Could you check a few things on this model? Use its own coordinates, in mm. A direction names the side the tool comes from. Round coordinates to 2 decimals unless told otherwise and drop trailing zeros. Write each loop counter-clockwise with the first axis right and the second up, starting at its lowest first coordinate (ties: lowest second). Pieces come first, ordered by that corner, then holes.
```python
from build123d import *

# Parameters (mm, degrees)
SKETCH1_W           = 54
SKETCH1_H           = 42
BOSS_EXTRUDE1_DEPTH = 40
BOSS_EXTRUDE2_DEPTH = 54
SKETCH12_W          = 20
SKETCH12_H          = 65.765371804
CUT_EXTRUDE5_DEPTH  = 157.508433956
SKETCH13_W          = 20
SKETCH13_H          = 20
CUT_EXTRUDE6_DEPTH  = 157.508433956
SKETCH14_W          = 7.9
SKETCH14_H          = 7.9
CUT_EXTRUDE7_DEPTH  = 20.2
BOSS_EXTRUDE3_DEPTH = 54
CUT_EXTRUDE8_DEPTH  = 54


with BuildPart() as part:
    # Sketch1 → Boss-Extrude1 (new body)
    with BuildSketch(Plane.XY):
        with Locations((27, 21)):
            Rectangle(SKETCH1_W, SKETCH1_H)
    extrude(amount=BOSS_EXTRUDE1_DEPTH)

    # Sketch5 → Boss-Extrude2 (add)
    with BuildSketch(Plane.ZY):
        Polygon((140.765371804, 42), (40, 42), (40, 0), (140.765371804, 27), align=None)
    extrude(amount=-BOSS_EXTRUDE2_DEPTH)

    # Sketch12 → Cut-Extrude5 (cut, through all)
    with BuildSketch(Plane(origin=(0, 42, 0), x_dir=(1, 0, 0), z_dir=(0, 1, 0))):
        with Locations((27, -67.882685902)):
            Rectangle(SKETCH12_W, SKETCH12_H)
    extrude(amount=-CUT_EXTRUDE5_DEPTH, mode=Mode.SUBTRACT)

    # Sketch13 → Cut-Extrude6 (cut, through all)
    with BuildSketch(Plane(origin=(0, 0, 0), x_dir=(-1, 0, 0), z_dir=(0, 0, -1))):
        with Locations((-27, 21)):
            Rectangle(SKETCH13_W, SKETCH13_H)
    extrude(amount=-CUT_EXTRUDE6_DEPTH, mode=Mode.SUBTRACT)

    # Sketch14 → Cut-Extrude7 (cut)
    with BuildSketch(Plane(origin=(0, 0, 0), x_dir=(-1, 0, 0), z_dir=(0, 0, -1))):
        with Locations((-45.25, 33.25)):
            Rectangle(SKETCH14_W, SKETCH14_H)
        with Locations((-45.25, 8.75)):
            Rectangle(SKETCH14_W, SKETCH14_H)
        with Locations((-8.75, 33.25)):
            Rectangle(SKETCH14_W, SKETCH14_H)
        with Locations((-8.75, 8.75)):
            Rectangle(SKETCH14_W, SKETCH14_H)
    extrude(amount=-CUT_EXTRUDE7_DEPTH, mode=Mode.SUBTRACT)

    # Sketch16 → Boss-Extrude3 (add)
    with BuildSketch(Plane(origin=(54, 0, 0), x_dir=(0, 0, -1), z_dir=(1, 0, 0))):
        Polygon((-140.765371804, 42), (-135.475562383, 72), (-87.112319758, 66.620193825), (-91.4535242, 42), align=None)
    extrude(amount=-BOSS_EXTRUDE3_DEPTH)

    # Sketch18 → Cut-Extrude8 (cut)
    with BuildSketch(Plane(origin=(54, 0, 0), x_dir=(0, 0, -1), z_dir=(1, 0, 0))):
        Polygon((-126.406728237, 70.991205567), (-135.475562383, 72), (-138.97204162, 52.170480871), (-121.632853281, 50.323309926), (-121.080075246, 55.292659626), (-126.9167299, 66.017283743), align=None)
        Polygon((-97.584499975, 67.785092966), (-98.201251534, 62.823277017), (-106.251724868, 53.643191009), (-106.804502902, 48.673841309), (-90.622534666, 46.712775836), (-87.112319758, 66.620193825), align=None)
    extrude(amount=-CUT_EXTRUDE8_DEPTH, mode=Mode.SUBTRACT)


solid = part.part
```
Q1. We'd pull the mould along Z, two halves only. Please class faces 5 (the flat face through (4.8, 33, 10)), 6 (the flat face through (27.378, 51.193, 106.524)), 7 (the flat face through (27, 37, 100.765)): pulls with the +Z half, pulls with the -Z half, needs draft (parallel to the pull), parting line crosses it, or undercut.
Q2. Imagine slicing it at D-D, the plane x = 44. Write out the boundary of the cut face in (y, z), then the cut area to 3 significant figures.
Q3. On a 3-axis mill with a long thin cutter (end or side, diameter ignored), from which of +Z, -Z, +X, -X, +Y, -Y can I reach the whole of each face in a straight line? I mean faces 1 (the flat face through (27.38, 58.3, 102.17)), 2 (the flat face through (27, 37, 35)), 3 (the flat face through (27.38, 52.77, 121.36)), 4 (the flat face through (9, 33, 20.2)). Say none if no direction works.
Q4. Imagine slicing it at C-C, the plane y = 40.5. Write out the boundary of the cut face in (x, z).
Q5. Imagine slicing it at B-B, the plane x = 34. Write out the boundary of the cut face in (y, z).
Q6. If I drill on L1, parallel to X at y = 5, z = 14.5; L2, parallel to Y at x = 45.5, z = 18.5; L3, parallel to X at y = 26, z = 123, over which ranges is the centre line in solid material (lowest first)?
Q7. Imagine slicing it at A-A, the plane z = 27. Write out the boundary of the cut face in (x, y).
Q8. I'm going to push flat-ended pins straight in: pin 1 Ø8.5 at (x, z) = (10.5, 5.5) entering from -Y; pin 2 Ø2.5 at (x, z) = (10, 11) entering from +Y; pin 3 Ø4 at (x, y) = (44.5, 8) entering from -Z; pin 4 Ø6 at (x, z) = (9, 71) entering from -Y. Where does each tip first touch, or does it pass through?
Results found:
1. face 5: needs draft
1. face 6: pulls with the -Z half
1. face 7: undercut
2. outline: (0, 0) - (4.8, 0) - (4.8, 20.2) - (12.7, 20.2) - (12.7, 0) - (29.3, 0) - (29.3, 20.2) - (37.2, 20.2) - (37.2, 0) - (42, 0) - (42, 91.45) - (46.71, 90.62) - (48.67, 106.8) - (53.64, 106.25) - (62.82, 98.2) - (67.79, 97.58) - (70.99, 126.41) - (66.02, 126.92) - (55.29, 121.08) - (50.32, 121.63) - (52.17, 138.97) - (42, 140.77) - (27, 140.77) - (0, 40) - close
2. area: 5,040 mm2
3. face 1: -Z, +X, -X
3. face 2: +Y, -Y
3. face 3: +X, -X
3. face 4: -Z
4. outline: (0, 0) - (54, 0) - (54, 140.77) - (0, 140.77) - close; hole (17, 35) - (37, 35) - (37, 100.77) - (17, 100.77) - close
5. outline: (0, 0) - (11, 0) - (11, 35) - (0, 35) - close; (31, 0) - (42, 0) - (42, 35) - (31, 35) - close; (31, 100.77) - (42, 100.77) - (42, 91.45) - (46.71, 90.62) - (48.67, 106.8) - (53.64, 106.25) - (62.82, 98.2) - (67.79, 97.58) - (70.99, 126.41) - (66.02, 126.92) - (55.29, 121.08) - (50.32, 121.63) - (52.17, 138.97) - (42, 140.77) - (31, 140.77) - close
6. L1: x = 0 to 4.8, 12.7 to 41.3, 49.2 to 54
6. L2: y = 0 to 4.8, 12.7 to 29.3, 37.2 to 42
6. L3: x = 0 to 17, 37 to 54
7. outline: (0, 0) - (54, 0) - (54, 42) - (0, 42) - close; hole (17, 11) - (37, 11) - (37, 31) - (17, 31) - close
8. pin 1: stops at y = 0
8. pin 2: stops at y = 42
8. pin 3: stops at z = 20.2
8. pin 4: stops at y = 7.5
